Read the model definition and answer for the solid it produces. Units are mm, in the model's axes. Face numbers are marked on the shaded views. A direction names the side the tool comes from. Coordinates: 2 decimals unless noted, no trailing zeros. Loops run counter-clockwise (first coordinate to the right, second up) from the corner with the lowest first, then second, coordinate; pieces in that order, holes last. Notation, with made-up numbers: (44, -24) -> (83, -24) arc R20 ccw to (83, 15) -> close; hole circle Ø7 at (11.25, 25). An arc over 180 degrees is marked (long way). Answer as CSV lines item,"result".
```python
from build123d import *

# Parameters (mm, degrees)
BOSS_EXTRUDE1_DEPTH = 3.175
SKETCH2_R           = 4.7625
BOSS_EXTRUDE2_DEPTH = 2.23012
SKETCH3_R           = 4.7625
SKETCH3_R_2         = 3.126994
BOSS_EXTRUDE3_DEPTH = 6.35
BOSS_EXTRUDE4_DEPTH = 1.5
FILLET1_1_64_R      = 0.396875
CHAMFER1_0_02_SIZE  = 0.508
CHAMFER2_0_005_SIZE = 0.127
CHAMFER3_0_01_SIZE  = 0.254


with BuildPart() as part:
    # Sketch1 → Boss-Extrude1 (new body)
    with BuildSketch(Plane(origin=(0, 0, 0), x_dir=(1, 0, 0), z_dir=(0, 1, 0))):
        Polygon((1.796425363, 3.1115), (-1.796425363, 3.1115), (-3.592850725, 0), (-1.796425363, -3.1115), (1.796425363, -3.1115), (3.592850725, 0), align=None)
    extrude(amount=BOSS_EXTRUDE1_DEPTH)

    # Sketch2 → Boss-Extrude2 (add)
    with BuildSketch(Plane(origin=(0, 3.175, 0), x_dir=(1, 0, 0), z_dir=(0, 1, 0))):
        with Locations(Location((0, 0, 0), (0, 0, 270))):
            Circle(SKETCH2_R)
    extrude(amount=BOSS_EXTRUDE2_DEPTH)

    # Sketch3 → Boss-Extrude3 (add)
    with BuildSketch(Plane(origin=(0, 5.40512, 0), x_dir=(1, 0, 0), z_dir=(0, 1, 0))):
        with Locations(Location((0, 0, 0), (0, 0, 270))):
            Circle(SKETCH3_R)
        with Locations(Location((0, 0, 0), (0, 0, 270))):
            Circle(SKETCH3_R_2, mode=Mode.SUBTRACT)
    extrude(amount=BOSS_EXTRUDE3_DEPTH)

    # Sketch4 → Boss-Extrude4 (add)
    with BuildSketch(Plane(origin=(0, 5.40512, 0), x_dir=(1, 0, 0), z_dir=(0, 1, 0))):
        with BuildLine():
            Line((-3.094445261, 0.45), (3.094445261, 0.45))
            ThreePointArc((3.094445261, 0.45), (3.126994, 0), (3.094445261, -0.45))
            Line((3.094445261, -0.45), (-3.094445261, -0.45))
            ThreePointArc((-3.094445261, -0.45), (-3.126994, 0), (-3.094445261, 0.45))
        make_face()
    extrude(amount=BOSS_EXTRUDE4_DEPTH)

    # Fillet1-1/64
    fillet1_1_64_edges = [part.edges().sort_by_distance(p)[0] for p in [
        (-2.694638044, 3.175, -1.55575),
        (3.592850725, 1.5875, 0),
        (1.796425363, 1.5875, 3.1115),
        (-1.796425363, 1.5875, 3.1115),
        (-3.592850725, 1.5875, 0),
        (-1.796425363, 1.5875, -3.1115),
        (1.796425363, 1.5875, -3.1115),
        (-2.694638044, 3.175, 1.55575),
        (0, 3.175, 3.1115),
        (2.694638044, 3.175, 1.55575),
        (0, 5.40512, -3.126994),
        (-2.045842635, 5.40512, 2.36487196),
        (-3.094445261, 6.15512, -0.45),
        (0, 5.40512, 0.45),
        (-3.094445261, 6.15512, 0.45),
        (3.094445261, 6.15512, 0.45),
        (0, 5.40512, -0.45),
        (3.094445261, 6.15512, -0.45),
        (2.694638044, 3.175, -1.55575),
        (0, 3.175, -3.1115),
    ]]
    fillet(fillet1_1_64_edges, radius=FILLET1_1_64_R)

    # Chamfer1-0.02
    chamfer1_0_02_edges = [part.edges().sort_by_distance(p)[0] for p in [
        (0, 3.175, -4.7625),
        (0, 11.75512, -4.7625),
        (0, 11.75512, -3.126994),
    ]]
    chamfer(chamfer1_0_02_edges, length=CHAMFER1_0_02_SIZE)

    # Chamfer2-0.005
    # the kernel refuses this chamfer: 0.127 mm, written as the material it takes off along each edge
    with BuildSketch(Plane(origin=(-2.595448418, 6.90512, -0.45), x_dir=(0, 0.027495876610587285, 0.9996219169112968), z_dir=(1, 0, 0)), Plane(origin=(2.595448418, 6.90512, 0.45), x_dir=(0, 0.027495876610587285, -0.9996219169112968), z_dir=(-1, 0, 0))) as chamfer2_0_005_piece_1:
        Polygon((CHAMFER2_0_005_SIZE * 0.999621916911, CHAMFER2_0_005_SIZE * 0.0274958766106), (-CHAMFER2_0_005_SIZE * 0.0274958766106, CHAMFER2_0_005_SIZE * 0.999621916911), (0, 0), align=None)
    extrude(amount=5.190896835, mode=Mode.SUBTRACT)
    with BuildSketch(Plane(origin=(-2.595448418, 6.90512, -0.846875), x_dir=(-0.4186703663111546, 0, -0.9081382738178606), z_dir=(0.9081382738178606, 0, -0.4186703663111546))) as chamfer2_0_005_piece_2_section:
        Polygon((0.396875 + CHAMFER2_0_005_SIZE, 0), (0.396875, -CHAMFER2_0_005_SIZE), (0.396875, 0), align=None)
    chamfer2_0_005_piece_2 = revolve(axis=Axis((-2.595448418, 6.90512, -0.846875), (0, 1, 0)), revolution_arc=155.249329417, mode=Mode.PRIVATE)
    chamfer2_0_005_piece_2 = chamfer2_0_005_piece_2 & Plane(origin=(0, 6.859082355, 0), x_dir=(0, 0, 1), z_dir=(0, -1, 0)) * Cylinder(3.126994, 3, mode=Mode.PRIVATE)
    add(chamfer2_0_005_piece_2, mode=Mode.SUBTRACT)
    with BuildSketch(Plane(origin=(-2.595448418, 6.90512, 0.846875), x_dir=(-0.41867036631116117, 0, 0.9081382738178575), z_dir=(0.9081382738178575, 0, 0.41867036631116117))) as chamfer2_0_005_piece_3_section:
        Polygon((0.396875, CHAMFER2_0_005_SIZE), (0.396875 + CHAMFER2_0_005_SIZE, 0), (0.396875, 0), align=None)
    chamfer2_0_005_piece_3 = revolve(axis=Axis((-2.595448418, 6.90512, 0.846875), (0, -1, 0)), revolution_arc=155.249329417, mode=Mode.PRIVATE)
    chamfer2_0_005_piece_3 = chamfer2_0_005_piece_3 & Plane(origin=(0, 6.859082356, 0), x_dir=(0, 0, 1), z_dir=(0, -1, 0)) * Cylinder(3.126994, 3, mode=Mode.PRIVATE)
    add(chamfer2_0_005_piece_3, mode=Mode.SUBTRACT)
    with BuildSketch(Plane(origin=(2.595448418, 6.90512, -0.846875), x_dir=(0.41867036631115895, 0, -0.9081382738178586), z_dir=(-0.9081382738178586, 0, -0.41867036631115895))) as chamfer2_0_005_piece_4_section:
        Polygon((0.396875 + CHAMFER2_0_005_SIZE, 0), (0.396875, CHAMFER2_0_005_SIZE), (0.396875, 0), align=None)
    chamfer2_0_005_piece_4 = revolve(axis=Axis((2.595448418, 6.90512, -0.846875), (0, -1, 0)), revolution_arc=155.249329417, mode=Mode.PRIVATE)
    chamfer2_0_005_piece_4 = chamfer2_0_005_piece_4 & Plane(origin=(0, 6.859082492, 0), x_dir=(0, 0, 1), z_dir=(0, -1, 0)) * Cylinder(3.126994, 3, mode=Mode.PRIVATE)
    add(chamfer2_0_005_piece_4, mode=Mode.SUBTRACT)
    with BuildSketch(Plane(origin=(2.595448418, 6.90512, 0.846875), x_dir=(0.41867036631115895, 0, 0.9081382738178586), z_dir=(-0.9081382738178586, 0, 0.41867036631115895))) as chamfer2_0_005_piece_5_section:
        Polygon((0.396875 + CHAMFER2_0_005_SIZE, 0), (0.396875, -CHAMFER2_0_005_SIZE), (0.396875, 0), align=None)
    chamfer2_0_005_piece_5 = revolve(axis=Axis((2.595448418, 6.90512, 0.846875), (0, 1, 0)), revolution_arc=155.249329417, mode=Mode.PRIVATE)
    chamfer2_0_005_piece_5 = chamfer2_0_005_piece_5 & Plane(origin=(0, 6.859082356, 0), x_dir=(0, 0, 1), z_dir=(0, -1, 0)) * Cylinder(3.126994, 3, mode=Mode.PRIVATE)
    add(chamfer2_0_005_piece_5, mode=Mode.SUBTRACT)

    # Chamfer3-0.01
    chamfer3_0_01_edges = [part.edges().sort_by_distance(p)[0] for p in [
        (2.694638044, 0, 1.55575),
        (2.694638044, 0, -1.55575),
        (0, 0, 3.1115),
        (-2.694638044, 0, 1.55575),
        (-2.694638044, 0, -1.55575),
        (0, 0, -3.1115),
        (1.765726974, 0, -3.058328832),
        (3.531453949, 0, 0),
        (-1.765726974, 0, -3.058328832),
        (-3.531453949, 0, 0),
        (-1.765726974, 0, 3.058328832),
        (1.765726974, 0, 3.058328832),
    ]]
    chamfer(chamfer3_0_01_edges, length=CHAMFER3_0_01_SIZE)


solid = part.part
```
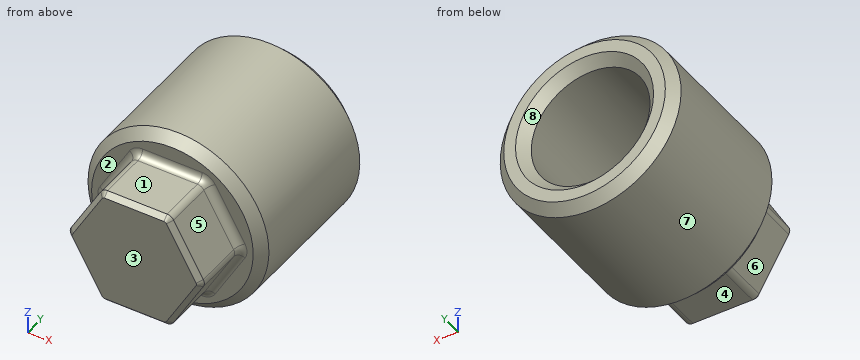
Q1. A cutting plane is placed at A-A, the plane y = 4. Write down the section's boundary in (x, z) (1 decimal), and give its area (3 significant figures).
Results:
outline,"circle Ø9.5 at (0, 0)"
area,"71.3 mm²"
Q2. Find the intervals of material crossed by probe 1 along X at (y, z) = (7.5, 0); probe 2 along Y at (x, z) = (-1.5, -3.75) (3 decimals); probe 3 along X at (y, z) = (10.5, 1.75), in increasing order. Write a range as [from, to].
Results:
probe 1,"x = [-4.76, -3.13], [3.13, 4.76]"
probe 2,"y = [3.175, 11.755]"
probe 3,"x = [-4.43, -2.59], [2.59, 4.43]"
Q3. Given pin 1 Ø4 at (x, z) = (0, 0) entering from +Y; pin 2 Ø1 at (x, z) = (-4, -3) entering from +Y; pin 3 Ø0.6 at (x, z) = (0, -2) entering from +Y, each flat-ended and moving along its own axis, determine where each tip first touches the part or whether it passes through.
Results:
pin 1,"stops at y = 6.91"
pin 2,"stops at y = 11.51"
pin 3,"stops at y = 5.41"
Q4. For the marked faces 1, 2, 3, 4 and 5, determine the directions among +Z, -Z, +X, -X, +Y, -Y from which every point of the face is accessible in a straight line to the end or side of a thin tool.
Results:
face 1,"+Z, +X, -X, -Y"
face 2,"-Y"
face 3,"+Z, -Z, +X, -X, -Y"
face 4,"-Z, +X, -X, -Y"
face 5,"+Z, +X, -Y"
Q5. A cutting plane is placed at B-B, the plane y = 11. Write down the section's boundary in (x, z) (1 decimal), and give its area (3 significant figures).
Results:
outline,"circle Ø9.5 at (0, 0); hole circle Ø6.3 at (0, 0)"
area,"40.5 mm²"
Q6. For a pull along X with two mould halves and no side action, classify the marked faces 6, 7 and 8 as pulls with the +X half, pulls with the -X half, needs draft (parallel to the pull), parting line crosses it, or undercut.
Results:
face 6,"pulls with the -X half"
face 7,"parting line crosses it"
face 8,"undercut"
